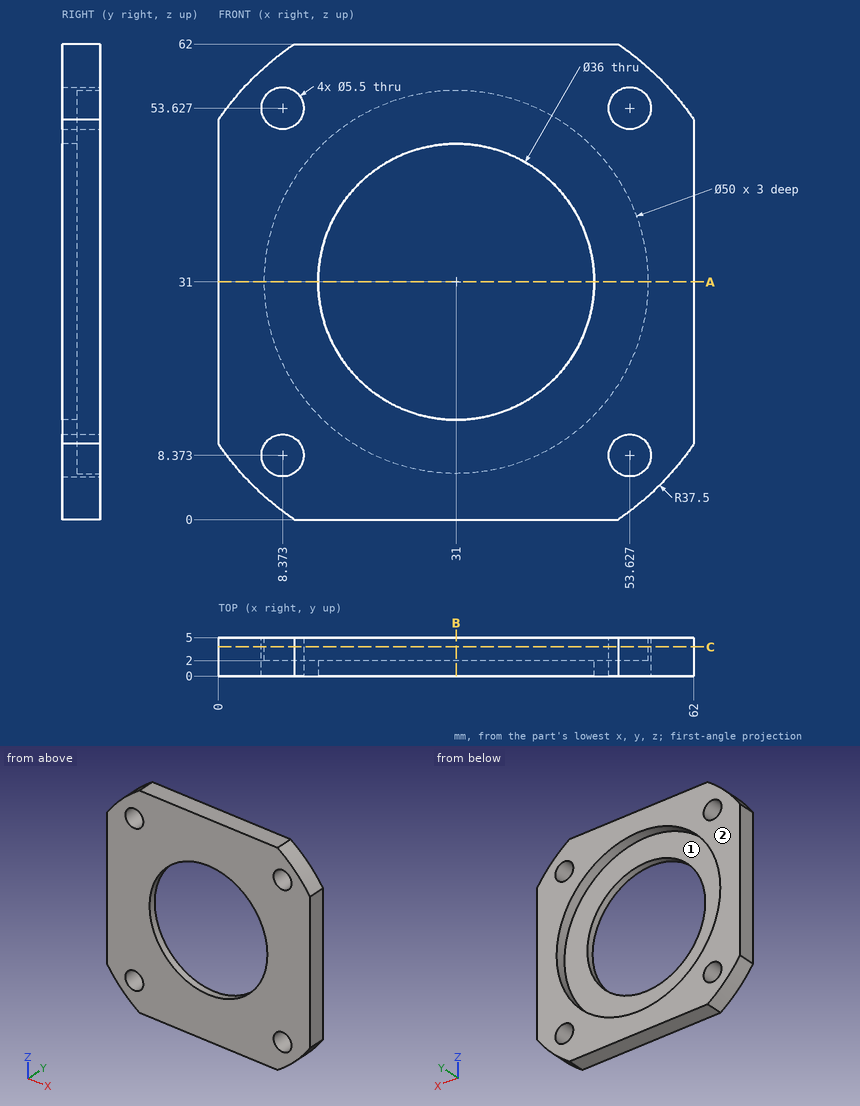
Source: three-view drawing plus pictorial views. Frame: mm from the lowest corner of the part. Round coordinates to 2 decimals unless told otherwise and drop trailing zeros. Order: outer loops, then holes, each group sorted by start corner. A loop starts at its lowest first (then second) coordinate and runs counter-clockwise, first axis right, second up. Notation, with made-up numbers: (-25, 20.5) - (26, 20.5) arc R20 cw to (26, 41.5) - close; hole circle Ø2 at (76.5, 3.25). An arc over 180 degrees is marked (long way). Answer in a Markdown table with one row per item.
Item 1: Section query A-A (z = 31). Return the cut outline in (x, y).
Model answer:
| item | result |
|---|---|
| outline | (0, 0) - (13, 0) - (13, 2) - (6, 2) - (6, 5) - (0, 5) - close; (49, 0) - (62, 0) - (62, 5) - (56, 5) - (56, 2) - (49, 2) - close |
Item 2: Pin query (flat end, axial travel): pin 1 (1 mm diameter, centred on y = 2, z = 8.5, fed in from -X). Return the tip coordinate at first contact, or that it passes through.
Model answer:
| item | result |
|---|---|
| pin 1 | stops at x = 0.63 |
Item 3: Mould query, pull axis Z, two halves, no side actions, for the marked faces 1 and 2. Classes: released by +Z, released by -Z, zero draft, split by the parting line, or undercut.
Model answer:
| item | result |
|---|---|
| face 1 | undercut |
| face 2 | zero draft |
Item 4: Section query B-B (x = 31). Return the cut outline in (y, z).
Model answer:
| item | result |
|---|---|
| outline | (0, 0) - (5, 0) - (5, 6) - (2, 6) - (2, 13) - (0, 13) - close; (0, 49) - (2, 49) - (2, 56) - (5, 56) - (5, 62) - (0, 62) - close |
Item 5: Section query C-C (y = 3.8). Return the cut outline in (x, z), then the cut area to 3 significant figures.
Model answer:
| item | result |
|---|---|
| outline | (0, 9.9) arc R37.5 ccw to (9.9, 0) - (52.1, 0) arc R37.5 ccw to (62, 9.9) - (62, 52.1) arc R37.5 ccw to (52.1, 62) - (9.9, 62) arc R37.5 ccw to (0, 52.1) - close; hole circle Ø5.5 at (8.37, 8.37); hole circle Ø5.5 at (8.37, 53.63); hole circle Ø50 at (31, 31); hole circle Ø5.5 at (53.63, 8.37); hole circle Ø5.5 at (53.63, 53.63) |
| area | 1,610 mm² |
Item 6: Line query: line 1 (Z direction, x = 54, y = 1.2); line 2 (Z direction, x = 31, y = 1.55); line 3 (Y direction, x = 10.5, z = 37.5). Output: solid intervals per line, ascending.
Model answer:
| item | result |
|---|---|
| line 1 | z = 1.38 to 5.65, 11.1 to 50.9, 56.35 to 60.62 |
| line 2 | z = 0 to 13, 49 to 62 |
| line 3 | y = 0 to 2 |
